Here's the drawing with two shaded views (mm, measured from the low corner). I have some questions. A direction names the side the tool comes from. Coordinates: 2 decimals unless noted, no trailing zeros. Loops run counter-clockwise (first coordinate to the right, second up) from the corner with the lowest first, then second, coordinate; pieces in that order, holes last. Notation, with made-up numbers: (73.25, 70) -> (84.25, 70) arc R13 ccw to (84.25, 90) -> close; hole circle Ø5 at (81.25, 82). An arc over 180 degrees is marked (long way). Answer as a JSON object with one key per item and string values. Group by question number.
Q1. I'm going to push flat-ended pins straight in: pin 1 (0.6 mm diameter, centred on y = 1.5, z = 19, fed in from +X); pin 2 (1.5 mm diameter, centred on x = 20, y = 2, fed in from +Z). Where does each tip first touch, or does it pass through?
Q2. I want a section at A-A on x = 25.4. Write out the boundary of the cut face in (y, z).
Q3. I need wall thicknesses on line 1 (Z direction, x = 6.35, y = 1.5); line 2 (Y direction, x = 25.25, z = 3.25); line 3 (X direction, y = 2.54, z = 3.5) (1 decimal). Which ranges of each line are inside material? Lowest first, please.
Q4. I want a section at D-D on z = 22.75. Write out the boundary of the cut face in (x, y).
Q5. I want a section at B-B on z = 3.5. Write out the boundary of the cut face in (x, y) (1 decimal).
Q6. On a 3-axis mill with a long thin cutter (end or side, diameter ignored), from which of +Z, -Z, +X, -X, +Y, -Y can I reach the whole of each face in a straight line? I mean the marked faces 1 and 2. Say none if no direction works.
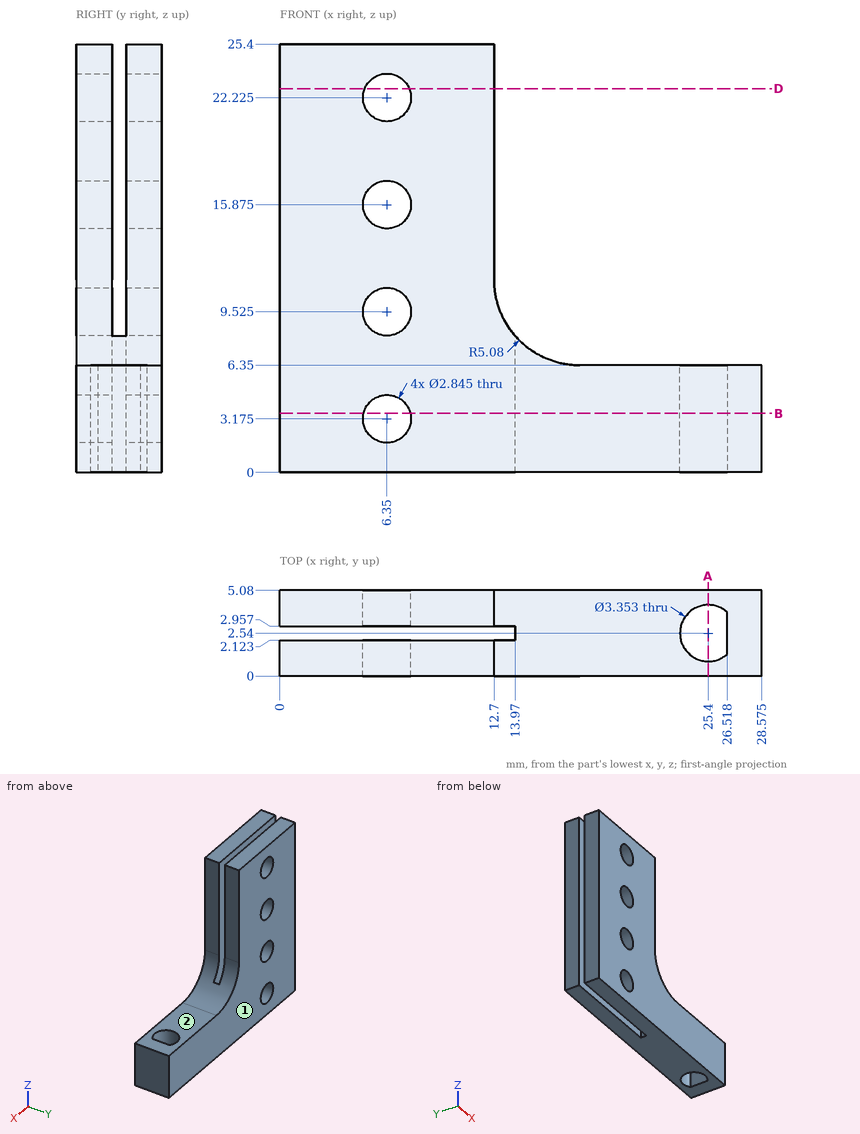
Result set:
{
 "1": {"pin 1": "stops at x = 12.7", "pin 2": "stops at z = 6.35"},
 "2": {"outline": "(0, 0) -> (0.86, 0) -> (0.86, 6.35) -> (0, 6.35) -> close; (4.22, 0) -> (5.08, 0) -> (5.08, 6.35) -> (4.22, 6.35) -> close"},
 "3": {"line 1": "z = 0 to 1.75, 4.6 to 8.1, 10.95 to 14.45, 17.3 to 20.8, 23.65 to 25.4", "line 2": "y = 0 to 0.87, 4.21 to 5.08", "line 3": "x = 14 to 23.7, 26.5 to 28.6"},
 "4": {"outline": "(0, 0) -> (5.03, 0) -> (5.03, 2.12) -> (0, 2.12) -> close; (0, 2.96) -> (5.03, 2.96) -> (5.03, 5.08) -> (0, 5.08) -> close; (7.67, 0) -> (12.7, 0) -> (12.7, 2.12) -> (7.67, 2.12) -> close; (7.67, 2.96) -> (12.7, 2.96) -> (12.7, 5.08) -> (7.67, 5.08) -> close"},
 "5": {"outline": "(0, 0) -> (5, 0) -> (5, 2.1) -> (0, 2.1) -> close; (0, 3) -> (5, 3) -> (5, 5.1) -> (0, 5.1) -> close; (7.7, 0) -> (28.6, 0) -> (28.6, 5.1) -> (7.7, 5.1) -> (7.7, 3) -> (14, 3) -> (14, 2.1) -> (7.7, 2.1) -> close; hole (26.5, 1.3) -> (26.5, 3.8) arc R1.7 ccw (long way) to start"},
 "6": {"face 1": "+Z, -Z, +X, -X, +Y", "face 2": "+Z, +X, +Y, -Y"}
}
